```python
from build123d import *

# Parameters (mm, degrees)
F0_R     = 45
F0_R_2   = 40
F1_DEPTH = 50
F0_R_3   = 50
F2_DEPTH = 100
F3_DEPTH = 5
F4_R     = 10
F5_DEPTH = 507.5


with BuildPart() as f1:
    # F0 (on Top) → F1 (new body)
    with BuildSketch(Plane.XY):
        Circle(F0_R)
        Circle(F0_R_2, mode=Mode.SUBTRACT)
    extrude(amount=F1_DEPTH)

    # F0 (on Top) → F2 (join)
    with BuildSketch(Plane.XY):
        Circle(F0_R_3)
        Circle(F0_R, mode=Mode.SUBTRACT)
    extrude(amount=F2_DEPTH)

    # F0 (on Top) → F3 (join)
    with BuildSketch(Plane.XY):
        Circle(F0_R_3)
        Circle(F0_R, mode=Mode.SUBTRACT)
        Circle(F0_R)
        Circle(F0_R_2, mode=Mode.SUBTRACT)
        Circle(F0_R_2)
    extrude(amount=F3_DEPTH)

    # F4
    f4_edges = [f1.edges().sort_by_distance(p)[0] for p in [
        (-50, 0, 0),
    ]]
    fillet(f4_edges, radius=F4_R)

    # F5 (add): a face of the model
    f5_faces = [f1.faces().sort_by_distance(p)[0] for p in [
        (-43.7272077939, 0, 50),
    ]]
    extrude(f5_faces, amount=F5_DEPTH)


solid = f1.part
```
Can you work these out from the model? Positions are in its coordinate system, mm. A direction names the side the tool comes from. Round coordinates to 2 decimals unless told otherwise and drop trailing zeros. Loops run counter-clockwise (first coordinate to the right, second up) from the corner with the lowest first, then second, coordinate; pieces in that order, holes last. Notation, with made-up numbers: M -27,-3.75 L -9,-3.75 A19 cw -9,21.25 Z; hole C 71.25,84 d6. An arc over 180 degrees is marked long. Answer in a Markdown table with one row per item.
1. If we section it at B-B, the plane z = 142: Please give me the cut outline in (x, y), plus the area to 3 significant figures.
Established:
| item | result |
|---|---|
| outline | C 0,0 d90; hole C 0,0 d80 |
| area | 1,340 mm² |
2. I'm going to push flat-ended pins straight in: pin 1 Ø6 at (x, z) = (-5, 473.5) entering from -Y; pin 2 Ø4 at (y, z) = (-15.5, 242) entering from +X; pin 3 Ø1 at (x, z) = (-33.5, 413) entering from -Y; pin 4 Ø12 at (x, y) = (37, -5.5) entering from +Z. Where does each tip first touch, or does it pass through?
Established:
| item | result |
|---|---|
| pin 1 | y = -44.96 |
| pin 2 | x = 42.93 |
| pin 3 | y = -30.59 |
| pin 4 | z = 557.5 |
3. Thinking about a two-plate mould opening in Y: for faces 1 (the face through (47.69, 15.02, 54.37)), 2 (the face through (-8.67, -39.05, 277.38)), 3 (the face through (-41, 19, 100)), which applies, pulls with the +Y half, pulls with the -Y half, needs draft (parallel to the pull), parting line crosses it, or undercut?
Established:
| item | result |
|---|---|
| face 1 | parting line crosses it |
| face 2 | undercut |
| face 3 | needs draft |
4. If we section it at A-A, the plane x = 0: Please give me the cut outline in (y, z).
Established:
| item | result |
|---|---|
| outline | M -50,10 A10 ccw -40,0 L 40,0 A10 ccw 50,10 L 50,100 L 45,100 L 45,557.5 L 40,557.5 L 40,5 L -40,5 L -40,557.5 L -45,557.5 L -45,100 L -50,100 Z |
5. On a 3-axis mill with a long thin cutter (end or side, diameter ignored), from which of +Z, -Z, +X, -X, +Y, -Y can I reach the whole of each face in a straight line? I mean faces 4 (the face through (-1, 1, 0)), 5 (the face through (20.765, -39.923, 325.548)). Say none if no direction works.
Established:
| item | result |
|---|---|
| face 4 | -Z, +X, -X, +Y, -Y |
| face 5 | +Z |
6. Please list where these lines run through material, in increasing order: line 1 (Y direction, x = 0, z = 432); line 2 (Z direction, x = -10, y = 4); line 3 (Y direction, x = -7.5, z = 368.5). Write a range as from..to.
Established:
| item | result |
|---|---|
| line 1 | -45..-40, 40..45 |
| line 2 | 0..5 |
| line 3 | -44.37..-39.29, 39.29..44.37 |
